Job drawing, mm, ordinate dimensions from the low corner. One solid piece. A direction names the side the tool comes from. Give positions to 0.01 mm unless a question says otherwise; leave off trailing zeros. Loops run counter-clockwise (first coordinate to the right, second up) from the corner with the lowest first, then second, coordinate; pieces in that order, holes last. Notation, with made-up numbers: (70, 77) - (106, 77) arc R32 cw to (106, 110) - close; hole circle Ø4 at (19, 73). An arc over 180 degrees is marked (long way). Answer as CSV lines item,"result". Start each with the question number.
Item 1: Saw through at C-C on z = 10.5. Give the cut face in (x, y), plus the area to 3 significant figures.
Item 2: Tool access for the marked faces 1 and 2: list every direction of +Z, -Z, +X, -X, +Y, -Y with a clear straight run to the whole face (end or side of a thin tool).
Item 3: Pin check, flat tips, straight feed: pin 1 (2.5 mm diameter, centred on x = 4.5, y = 4.5, fed in from -Z); pin 2 (1.2 mm diameter, centred on x = 31, y = 30.5, fed in from -Z). Stop position of each tip, or through.
Item 4: Saw through at D-D on x = 26. Give the cut face in (y, z).
Item 5: Saw through at A-A on x = 17.6. Give the cut face in (y, z).
Item 6: Drill centre lines: L1, parallel to X at y = 4.6, z = 25.25; L2, parallel to Y at x = 4, z = 25. Where is each one in solid material? Low to high. Write a range as from..to.
Item 7: Saw through at B-B on y = 30.6. Give the cut face in (x, z).
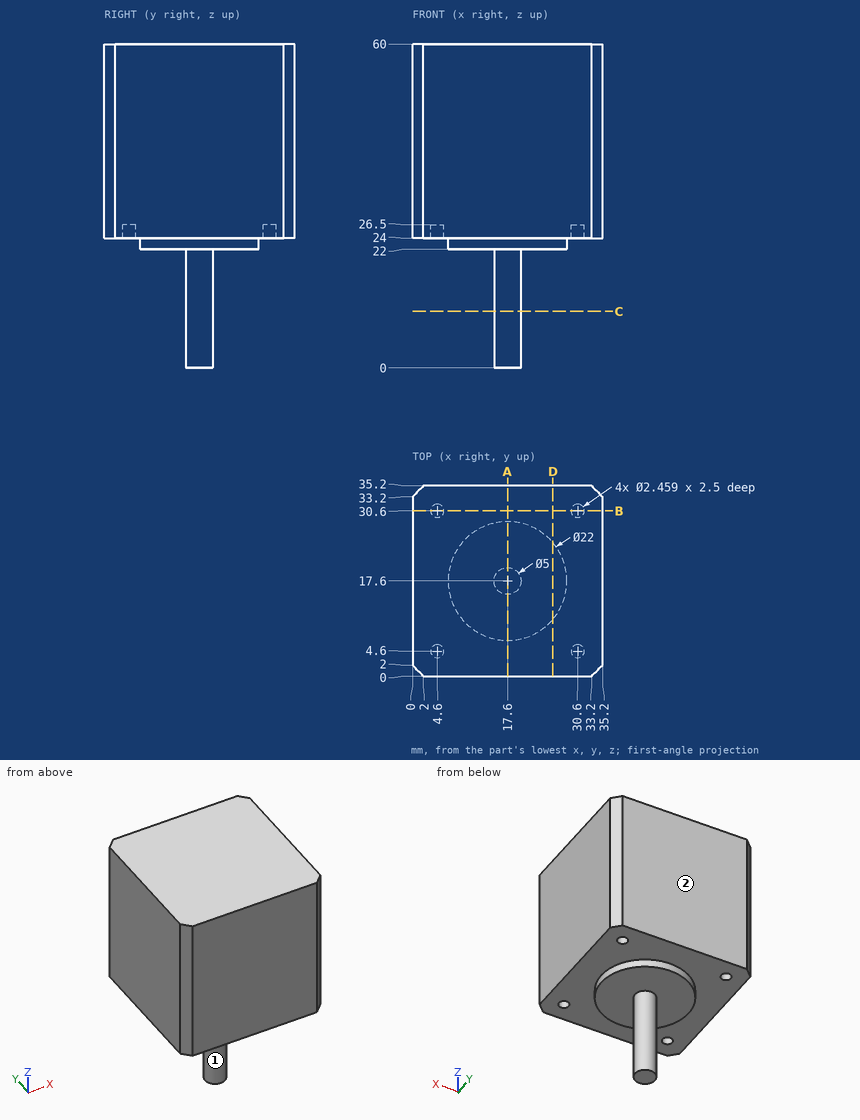
Responses:
1,outline,"circle Ø5 at (17.6, 17.6)"
1,area,"19.6 mm2"
2,face 1,"-Z"
2,face 2,"+Z, -Z, +X, -X, +Y"
3,pin 1,"z = 24"
3,pin 2,"z = 26.5"
4,outline,"(0, 24) - (10.5, 24) - (10.5, 22) - (24.7, 22) - (24.7, 24) - (35.2, 24) - (35.2, 60) - (0, 60) - close"
5,outline,"(0, 24) - (6.6, 24) - (6.6, 22) - (15.1, 22) - (15.1, 0) - (20.1, 0) - (20.1, 22) - (28.6, 22) - (28.6, 24) - (35.2, 24) - (35.2, 60) - (0, 60) - close"
6,L1,"0..3.37, 5.83..29.37, 31.83..35.2"
6,L2,"0..3.53, 5.67..29.53, 31.67..35.2"
7,outline,"(0, 24) - (3.37, 24) - (3.37, 26.5) - (5.83, 26.5) - (5.83, 24) - (29.37, 24) - (29.37, 26.5) - (31.83, 26.5) - (31.83, 24) - (35.2, 24) - (35.2, 60) - (0, 60) - close"
